Work out the finished part from the listing and answer in its coordinate system (mm). Give positions to 0.01 mm unless a question says otherwise; leave off trailing zeros. Order: outer loops, then holes, each group sorted by start corner. A loop starts at its lowest first (then second) coordinate and runs counter-clockwise, first axis right, second up. Notation, with made-up numbers: (82, -5.5) -> (107, -5.5) arc R27 cw to (107, 27.5) -> close; hole circle Ø10 at (-27, 59). An arc over 180 degrees is marked (long way). Use a Markdown table: item, result. Add a question column.
Autodesk Inventor part; units mm, degrees
ref_plane "Arbeitsebene1" through (-7.5, 0, 0) normal (1, 0, 0) x (0, 1, 0)
ref_plane "Arbeitsebene2" through (7.5, 0, 0) normal (1, 0, 0) x (0, 1, 0)
ref_plane "XZ Plane" through (0, 0, 0) normal (0, 1, 0) x (-1, 0, 0)
sketch "Skizze1" plane through (0, 0, 0) normal (0, 1, 0) x (-1, 0, 0)
  circle A0 centre (0, 0) radius 12.5
  dimension "d0" = 25
extrude "Extrusion1" add sketch "Skizze1" along normal blind 765.83
ref_plane "Arbeitsebene1" through (-7.5, 0, 0) normal (1, 0, 0) x (0, 1, 0)
ref_plane "Arbeitsebene2" through (7.5, 0, 0) normal (1, 0, 0) x (0, 1, 0)
sketch "Skizze4" plane through (0, 765.83, 0) normal (0, 1, 0) x (1, 0, 0)
  line L0 (3.5, -16) -> (-3.5, -16)
  line L1 (-3.5, -16) -> (-3.5, -6)
  line L2 (-3.5, -6) -> (3.5, -6)
  line L3 (3.5, -6) -> (3.5, -16)
  line L4 (0, 18.2) -> (0, -21.7) construction
  line L5 (-17.5, 0) -> (17.5, 0) construction
  dimension "d15" = 6
  dimension "d16" = 10
  dimension "d17" = 7
extrude "Extrusion4" cut sketch "Skizze4" against normal blind 12
sketch "Skizze5" plane through (0, 0, 0) normal (0, -1, 0) x (1, 0, 0)
  line L0 (-3.8549, 16) -> (3.1451, 16)
  line L1 (3.1451, 16) -> (3.1451, 6)
  line L2 (3.1451, 6) -> (-3.8549, 6)
  line L3 (-3.8549, 6) -> (-3.8549, 16)
  line L4 (-17.5, 0) -> (17.5, 0) construction
  dimension "d20" = 6
  dimension "d21" = 10
  dimension "d22" = 7
extrude "Extrusion5" cut sketch "Skizze5" against normal blind 12
equation "\"Wellensdurchmesser\" = 35"
equation "\"Wellenlänge\" = 724.33"
properties part number "Welle"
1) Straight lines are drawn through the part: line 1 (X direction, y = 207, z = 0.5); line 2 (Z direction, x = 0, y = 131); line 3 (Y direction, x = 0, z = 9). For each, find the intervals that lie inside material, in ascending order.
2) The part is cut by section A-A, the plane y = 434. Determine the outline of the cut face in (x, z).
3) Flat-ended cylindrical pins translate along their axes: pin 1 (2 mm diameter, centred on x = -1, z = 10, fed in from +Y); pin 2 (4 mm diameter, centred on x = 1.5, z = 7.5, fed in from +Y); pin 3 (10 mm diameter, centred on y = 560, z = 6.5, fed in from +X); pin 4 (5.5 mm diameter, centred on x = -0.5, y = 760, fed in from +Z). Find the tip coordinate at first contact, or state that the pin passes through.
A:
| question | item | result |
|---|---|---|
| 1 | line 1 | -12.49 to 12.49 |
| 1 | line 2 | -12.5 to 12.5 |
| 1 | line 3 | 12 to 753.83 |
| 2 | outline | circle Ø25 at (0, 0) |
| 3 | pin 1 | y = 753.83 |
| 3 | pin 2 | y = 765.83 |
| 3 | pin 3 | x = 12.41 |
| 3 | pin 4 | z = 6 |
